```python
from build123d import *

# Parameters (mm, degrees)
SKETCH1_W           = 25
SKETCH1_H           = 25
BOSS_EXTRUDE1_DEPTH = 1
SKETCH2_W           = 23
SKETCH2_H           = 23
BOSS_EXTRUDE2_DEPTH = 3
SHELL1_START        = -3
SHELL1_OUTLINE_W    = 21
SHELL1_OUTLINE_H    = 21
SHELL1_DEPTH        = 3
SKETCH3_W           = 7.5
SKETCH3_H           = 4
CUT_EXTRUDE1_DEPTH  = 10


# Read off the part's stored shape, not the designer's step: Shell1
with BuildPart() as part:
    # Sketch1 → Boss-Extrude1 (new body)
    with BuildSketch(Plane.XY):
        Rectangle(SKETCH1_W, SKETCH1_H)
    extrude(amount=BOSS_EXTRUDE1_DEPTH)

    # Sketch2 → Boss-Extrude2 (add)
    with BuildSketch(Plane(origin=(0, 0, 0), x_dir=(-1, 0, 0), z_dir=(0, 0, -1))):
        Rectangle(SKETCH2_W, SKETCH2_H)
    extrude(amount=BOSS_EXTRUDE2_DEPTH)

    # Shell1 outline → Shell1 (cut)
    with BuildSketch(Plane.XY.offset(SHELL1_START)):
        Rectangle(SHELL1_OUTLINE_W, SHELL1_OUTLINE_H)
    extrude(amount=SHELL1_DEPTH, mode=Mode.SUBTRACT)

    # Sketch3 → Cut-Extrude1 (cut)
    with BuildSketch(Plane(origin=(0, 0, 0), x_dir=(-1, 0, 0), z_dir=(0, 0, -1))):
        Rectangle(SKETCH3_W, SKETCH3_H)
    extrude(amount=-CUT_EXTRUDE1_DEPTH, mode=Mode.SUBTRACT)


solid = part.part
```
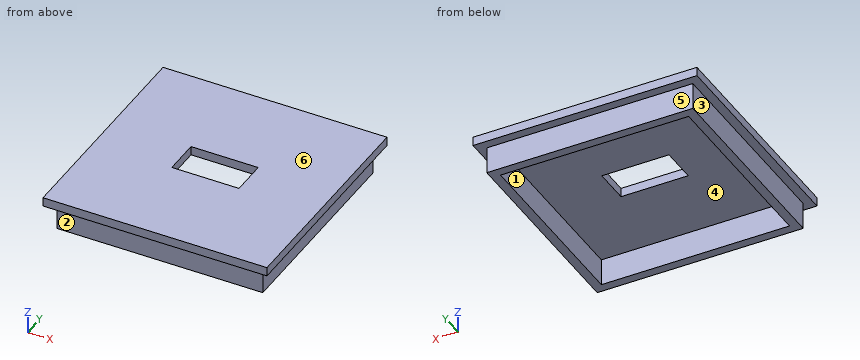
Can you work these out from the model? Positions are in its coordinate system, mm. Face numbers are marked on the shaded views. A direction names the side the tool comes from. Round coordinates to 2 decimals unless told otherwise and drop trailing zeros. Loops run counter-clockwise (first coordinate to the right, second up) from the corner with the lowest first, then second, coordinate; pieces in that order, holes last. Notation, with made-up numbers: M 22,-32.5 L 79,-32.5 A11 cw 79,-26.5 Z; hole C 67.5,32 d9. An arc over 180 degrees is marked long. Answer in a Markdown table with one row per item.
1. Please list where these lines run through material, in increasing order: line 1 (X direction, y = -4, z = -0.1); line 2 (Y direction, x = -1.25, z = 0.2). Write a range as from..to.
Established:
| item | result |
|---|---|
| line 1 | -11.5..-10.5, 10.5..11.5 |
| line 2 | -12.5..-2, 2..12.5 |
2. If we section it at C-C, the plane y = -0.5: Please give me the cut outline in (x, z), plus the area to 3 significant figures.
Established:
| item | result |
|---|---|
| outline | M -12.5,0 L -11.5,0 L -11.5,-3 L -10.5,-3 L -10.5,0 L -3.75,0 L -3.75,1 L -12.5,1 Z; M 3.75,0 L 10.5,0 L 10.5,-3 L 11.5,-3 L 11.5,0 L 12.5,0 L 12.5,1 L 3.75,1 Z |
| area | 23.5 mm² |
3. I'm going to push flat-ended pins straight in: pin 1 Ø1.5 at (x, z) = (0, -2) entering from +Y; pin 2 Ø2 at (x, z) = (-6, -0.5) entering from -Y; pin 3 Ø1.5 at (y, z) = (-3, -1.5) entering from -X; pin 4 Ø1.5 at (x, z) = (4.5, -1.5) entering from -Y. Where does each tip first touch, or does it pass through?
Established:
| item | result |
|---|---|
| pin 1 | y = 11.5 |
| pin 2 | y = -12.5 |
| pin 3 | x = -11.5 |
| pin 4 | y = -11.5 |
4. If we section it at B-B, the plane z = 0.3: Please give me the cut outline in (x, y).
Established:
| item | result |
|---|---|
| outline | M -12.5,-12.5 L 12.5,-12.5 L 12.5,12.5 L -12.5,12.5 Z; hole M -3.75,-2 L 3.75,-2 L 3.75,2 L -3.75,2 Z |
5. On a 3-axis mill with a long thin cutter (end or side, diameter ignored), from which of +Z, -Z, +X, -X, +Y, -Y can I reach the whole of each face in a straight line? I mean the marked faces 4, 5 and 6. Say none if no direction works.
Established:
| item | result |
|---|---|
| face 4 | -Z |
| face 5 | -Z, +X, -X, +Y |
| face 6 | +Z, +X, -X, +Y, -Y |
6. If we section it at A-A, the plane x = 0: Please give me the cut outline in (y, z).
Established:
| item | result |
|---|---|
| outline | M -12.5,0 L -11.5,0 L -11.5,-3 L -10.5,-3 L -10.5,0 L -2,0 L -2,1 L -12.5,1 Z; M 2,0 L 10.5,0 L 10.5,-3 L 11.5,-3 L 11.5,0 L 12.5,0 L 12.5,1 L 2,1 Z |
7. Thinking about a two-plate mould opening in X: for the marked faces 1, 2 and 3, which applies, pulls with the +X half, pulls with the -X half, needs draft (parallel to the pull), parting line crosses it, or undercut?
Established:
| item | result |
|---|---|
| face 1 | undercut |
| face 2 | needs draft |
| face 3 | pulls with the -X half |
8. If we section it at D-D, the plane y = -6.5: Please give me the cut outline in (x, z), plus the area to 3 significant figures.
Established:
| item | result |
|---|---|
| outline | M -12.5,0 L -11.5,0 L -11.5,-3 L -10.5,-3 L -10.5,0 L 10.5,0 L 10.5,-3 L 11.5,-3 L 11.5,0 L 12.5,0 L 12.5,1 L -12.5,1 Z |
| area | 31.0 mm² |
